Answer from the drawing. Dimensions are ordinates in mm from the lowest x, y and z of the part. Give positions to 0.01 mm unless a question says otherwise; leave off trailing zeros. Write each loop counter-clockwise with the first axis right and the second up, starting at its lowest first coordinate (ties: lowest second). Pieces come first, ordered by that corner, then holes. Notation, with made-up numbers: (65, 12.5) - (92, 12.5) arc R19 ccw to (92, 49.5) - close; hole circle Ø10 at (-16, 4). An arc over 180 degrees is marked (long way). Write item = value, one per line.
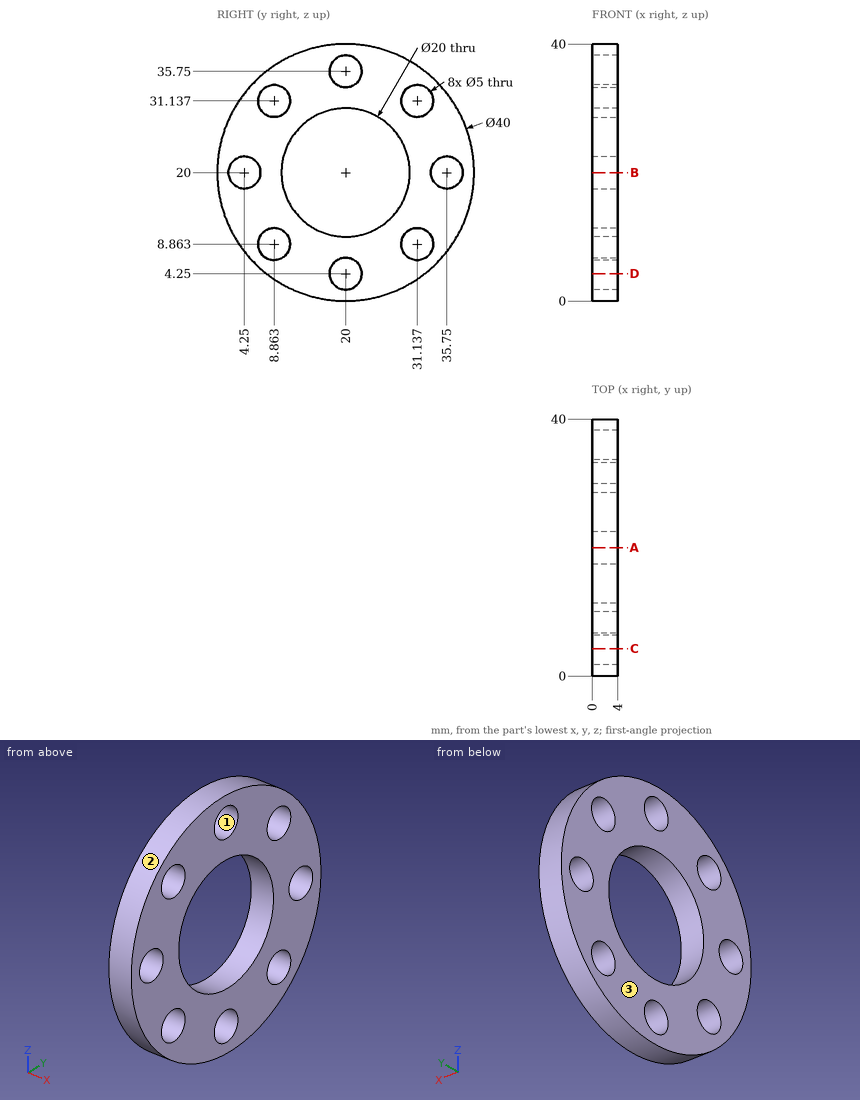
1. For a pull along Z with two mould halves and no side action, classify the marked faces 1, 2 and 3 as pulls with the +Z half, pulls with the -Z half, needs draft (parallel to the pull), parting line crosses it, or undercut.
Solution:
face_1 = undercut
face_2 = parting line crosses it
face_3 = needs draft
2. Straight lines are drawn through the part: line 1 (Z direction, x = 3, y = 20); line 2 (Y direction, x = 3, z = 33); line 3 (Y direction, x = 2.85, z = 9.5). For each, find the intervals that lie inside material, in ascending order.
Solution:
line_1 = 0 to 1.75, 6.75 to 10, 30 to 33.25, 38.25 to 40
line_2 = 4.8 to 7.2, 10.53 to 29.47, 32.8 to 35.2
line_3 = 2.98 to 6.45, 11.28 to 28.72, 33.55 to 37.02
3. Find section A-A, the plane y = 20. Give the vertices of the cut face in (x, z).
Solution:
outline = (0, 0) - (4, 0) - (4, 1.75) - (0, 1.75) - close; (0, 6.75) - (4, 6.75) - (4, 10) - (0, 10) - close; (0, 30) - (4, 30) - (4, 33.25) - (0, 33.25) - close; (0, 38.25) - (4, 38.25) - (4, 40) - (0, 40) - close
4. Given pin 1 (1 mm diameter, centred on x = 1, y = 26, fed in from +Z); pin 2 (1.5 mm diameter, centred on x = 3, y = 28.5, fed in from +Z); pin 3 (1 mm diameter, centred on x = 1, y = 35.5, fed in from -Z), each flat-ended and moving along its own axis, determine where each tip first touches the part or whether it passes through.
Solution:
pin_1 = 39.23
pin_2 = 38.44
pin_3 = 6.77
5. Find section C-C, the plane y = 4.25. Give the vertices of the cut face in (x, z).
Solution:
outline = (0, 7.67) - (4, 7.67) - (4, 17.5) - (0, 17.5) - close; (0, 22.5) - (4, 22.5) - (4, 32.33) - (0, 32.33) - close
